from build123d import *

# Parameters (mm, degrees)
F0_W     = 203.2
F0_H     = 152.4
F1_DEPTH = 25.4
F3_DEPTH = 38.1
F4_W     = 203.2
F4_H     = 51.9680035462
F5_DEPTH = 50.8


# Not quite as in the source:
# - a feature names something its author has since deleted; it is built from what else it names


with BuildPart() as f1:
    # F0 (on Front) → F1 (new body)
    with BuildSketch(Plane.XZ):
        with Locations((21.5330033839, 24.2319964538)):
            Rectangle(F0_W, F0_H)
    extrude(amount=F1_DEPTH)

    # F2 (on face) → F3 (join)
    with BuildSketch(Plane.XZ.offset(25.4)):
        Polygon((-29.2669966161, 32.6819717884), (-29.2669966161, 100.4319964538), (-80.0669966161, 100.4319964538), (-80.0669966161, -51.9680035462), (123.1330033839, -51.9680035462), (123.1330033839, 100.4319964538), (72.3330033839, 100.4319964538), (72.3330033839, 32.6819717884), align=None)
    extrude(amount=F3_DEPTH)

    # F4 (on face) → F5 (join)
    with BuildSketch(Plane.XZ.offset(63.5)):
        with Locations((21.5330033839, -25.9840017731)):
            Rectangle(F4_W, F4_H)
    extrude(amount=F5_DEPTH)


solid = f1.part
The listing builds one solid part. Answer for the finished solid, in the listing's coordinates (mm). A direction names the side the tool comes from. Coordinates: 2 decimals unless noted, no trailing zeros. Write each loop counter-clockwise with the first axis right and the second up, starting at its lowest first coordinate (ties: lowest second). Pieces come first, ordered by that corner, then holes. Notation, with made-up numbers: (-37, -3) -> (-33, -3) arc R14 ccw to (-33, 22) -> close; hole circle Ø1 at (55.5, -28). An arc over 180 degrees is marked (long way). One line per question, with ' | ' between items.
1. Section B-B (z = 90.5) is taken. Determine the outline of the cut face in (x, y).
Verdict:
outline: (-80.07, -63.5) -> (-29.27, -63.5) -> (-29.27, -25.4) -> (72.33, -25.4) -> (72.33, -63.5) -> (123.13, -63.5) -> (123.13, 0) -> (-80.07, 0) -> close
2. For a pull along X with two mould halves and no side action, classify faces 4 (the flat face through (-80.067, -44, 6)), 5 (the flat face through (72.333, -44, 67)), 6 (the flat face through (20, -114.3, -26)) as released by +X, released by -X, zero draft, split by the parting line, or undercut.
Verdict:
face 4: released by -X | face 5: undercut | face 6: zero draft
3. Given pin 1 Ø10 at (x, y) = (68, -85.5) entering from +Z; pin 2 Ø1.5 at (x, z) = (63.5, -7.5) entering from +Y; pin 3 Ø11.5 at (x, y) = (26, -46.5) entering from +Z, each flat-ended and moving along its own axis, determine where each tip first touches the part or whether it passes through.
Verdict:
pin 1: stops at z = 0 | pin 2: stops at y = 0 | pin 3: stops at z = 32.68
4. Section D-D (z = 17) is taken. Determine the outline of the cut face in (x, y), and give its area (3 significant figures).
Verdict:
outline: (-80.07, -63.5) -> (123.13, -63.5) -> (123.13, 0) -> (-80.07, 0) -> close | area: 12,900 mm^2
5. Straight lines are drawn through the part: line 1 (X direction, y = -53, z = 49.5); line 2 (Y direction, x = 101.5, z = 44.5); line 3 (Z direction, x = -68, y = -74). For each, find the intervals that lie inside material, in ascending order.
Verdict:
line 1: x = -80.07 to -29.27, 72.33 to 123.13 | line 2: y = -63.5 to 0 | line 3: z = -51.97 to 0
6. Section A-A (y = -48) is taken. Determine the outline of the cut face in (x, z).
Verdict:
outline: (-80.07, -51.97) -> (123.13, -51.97) -> (123.13, 100.43) -> (72.33, 100.43) -> (72.33, 32.68) -> (-29.27, 32.68) -> (-29.27, 100.43) -> (-80.07, 100.43) -> close
7. Which of the six approach directions +Z, -Z, +X, -X, +Y, -Y give full straight-line access (tool end or side, diameter ignored) to faces 1 (the flat face through (-29.267, -44, 66)), 2 (the flat face through (20, -56, -51.968)), 3 (the flat face through (20, -63.5, 29))?
Verdict:
face 1: +Z, -Y | face 2: -Z, +X, -X, +Y, -Y | face 3: +Z, +X, -X, -Y
8. Section C-C (x = 103.5) is taken. Determine the outline of the cut face in (y, z).
Verdict:
outline: (-114.3, -51.97) -> (0, -51.97) -> (0, 100.43) -> (-63.5, 100.43) -> (-63.5, 0) -> (-114.3, 0) -> close
